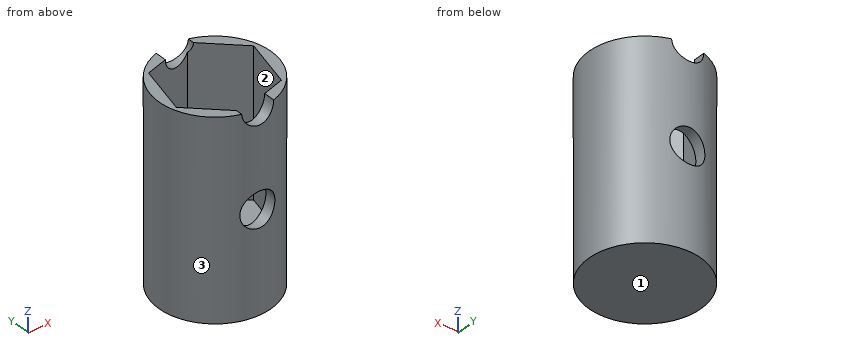
```python
from build123d import *

# Parameters (mm, degrees)
F0_R      = 27.5
F1_DEPTH  = 25
F1_FACE_R = 27.5
F2_DEPTH  = 71.1
F4_DEPTH  = 71.7
F6_R      = 7.831507
F7_DEPTH  = 739.1
F8_R      = 8.573523
F9_DEPTH  = 106


with BuildPart() as f1:
    # F0 (on Top) → F1 (new body)
    with BuildSketch(Plane.XY):
        Circle(F0_R)
    extrude(amount=F1_DEPTH)

    # F1_face (on face) → F2 (join)
    with BuildSketch(Plane.XY.offset(25)):
        Circle(F1_FACE_R)
    extrude(amount=F2_DEPTH)

    # F3 (on face) → F4 (cut)
    with BuildSketch(Plane.XY.offset(96.1)):
        Polygon((-6.105004, -24.826832), (18.448165, -17.700505), (24.553169, 7.126327), (6.105004, 24.826832), (-18.448165, 17.700505), (-24.553169, -7.126327), align=None)
    extrude(amount=-F4_DEPTH, mode=Mode.SUBTRACT)

    # F6 (on offset) → F7 (cut)
    with BuildSketch(Plane.XZ.offset(50)):
        with Locations((0, 96.259676)):
            Circle(F6_R)
    extrude(amount=-F7_DEPTH, mode=Mode.SUBTRACT)

    # F8 (on offset) → F9 (cut)
    with BuildSketch(Plane.XZ.offset(50)):
        with Locations((0, 49.162731)):
            Circle(F8_R)
    extrude(amount=-F9_DEPTH, mode=Mode.SUBTRACT)


solid = f1.part
```
The model under review builds one solid part; all positions refer to its coordinate system, in mm. Face numbers are marked on the shaded views. Give positions to 0.01 mm unless a question says otherwise; leave off trailing zeros. Write each loop counter-clockwise with the first axis right and the second up, starting at its lowest first coordinate (ties: lowest second). Pieces come first, ordered by that corner, then holes.
(1) Consider section D-D, the plane x = 12. Give the boundary of the cut face in (y, z).
(2) Consider section A-A, the plane z = 83. Give the boundary of the cut face in (x, y) (1 decimal), and give its area (3 significant figures).
(3) To check wall thickness, follow L1, parallel to Y at x = -2, z = 86; L2, parallel to X at y = 15, z = 71; L3, parallel to X at y = 6, z = 92.5. State the ranges of each line that lie inside material, in increasing order.
(4) Consider section B-B, the plane x = 0. Give the boundary of the cut face in (y, z), and give its area (3 significant figures).
(5) The part is to be moulded in two halves that separate along X. For the marked faces 1, 2 and 3, say which applies: released by +X, released by -X, zero draft, split by the parting line, or undercut.
(6) Consider section C-C, the plane y = -22. Give the boundary of the cut face in (x, z), and give its area (3 significant figures).
(7) For P1, Ø3, axis at y = 5.5, z = 85.5, coming from the -X side; P2, Ø2, axis at x = -6, y = -21, coming from the -Z side; P3, Ø10, axis at x = -11, z = 49, coming from the -Y side; P4, Ø3, axis at y = 7.5, z = 54.5, coming from the -X side, all flat-tipped, find the tip position at first contact; note any pin that passes through.
Returned:
1. outline: (-24.74, 0) - (24.74, 0) - (24.74, 96.1) - (19.17, 96.1) - (19.17, 24.4) - (-19.57, 24.4) - (-19.57, 96.1) - (-24.74, 96.1) - close
2. outline: circle Ø55 at (0, 0); hole (-24.6, -7.1) - (-6.1, -24.8) - (18.4, -17.7) - (24.6, 7.1) - (6.1, 24.8) - (-18.4, 17.7) - close
2. area: 678 mm2
3. L1: y = -27.43 to -23.64, 22.47 to 27.43
3. L2: x = -23.05 to -19.11, 16.35 to 23.05
3. L3: x = -26.84 to -21.33, 24.28 to 26.84
4. outline: (-27.5, 0) - (27.5, 0) - (27.5, 40.59) - (23.05, 40.59) - (23.05, 24.4) - (-23.05, 24.4) - (-23.05, 40.59) - (-27.5, 40.59) - close; (-27.5, 57.74) - (-23.05, 57.74) - (-23.05, 88.43) - (-27.5, 88.43) - close; (23.05, 57.74) - (27.5, 57.74) - (27.5, 88.43) - (23.05, 88.43) - close
4. area: 1,760 mm2
5. face 1: zero draft
5. face 2: undercut
5. face 3: split by the parting line
6. outline: (-16.5, 0) - (16.5, 0) - (16.5, 96.1) - (7.83, 96.1) arc R7.83 cw to (3.63, 89.32) - (3.63, 56.93) arc R8.57 cw to (3.63, 41.4) - (3.63, 24.4) - (-9.05, 24.4) - (-9.05, 96.1) - (-16.5, 96.1) - close
6. area: 2,190 mm2
7. P1: stops at x = -27.21
7. P2: stops at z = 0
7. P3: stops at y = -26.41
7. P4: stops at x = -26.84
